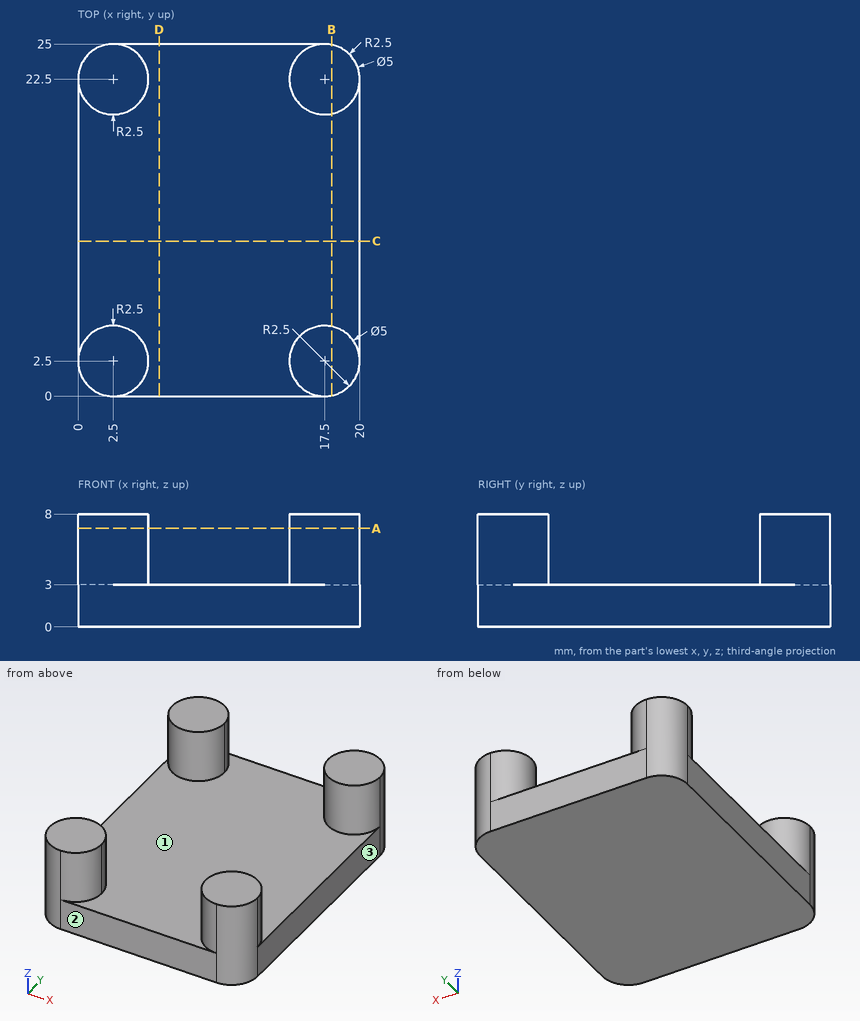
Study the drawing (mm; zero at the part's minimum x, y, z) and answer. Coordinates: 2 decimals unless noted, no trailing zeros. Write each loop counter-clockwise with the first axis right and the second up, starting at its lowest first coordinate (ties: lowest second). Pieces come first, ordered by that corner, then holes.
Q1. A cutting plane is placed at C-C, the plane y = 11. Give the vertices of the cut face in (x, z).
Q2. A cutting plane is placed at B-B, the plane x = 18. Give the vertices of the cut face in (y, z), then the cut area to 3 significant figures.
Q3. Determine the mould class of the marked faces 1, 2 and 3 for opening direction Y: released by +Y, released by -Y, zero draft, split by the parting line, or undercut.
Q4. Each of these flat-tipped pins is pushed along its axis until it touches: pin 1 Ø1 at (x, y) = (5, 21) entering from +Z; pin 2 Ø1 at (x, z) = (11, 4.5) entering from -Y; pin 3 Ø3 at (x, y) = (11, 5.5) entering from +Z. Where does it stop, or does it pass through?
Q5. A cutting plane is placed at D-D, the plane x = 5.75. Give the vertices of the cut face in (y, z).
Q6. A cutting plane is placed at A-A, the plane z = 7. Give the vertices of the cut face in (x, y), then the cut area to 3 significant figures.
Q7. Find the intervals of material crossed by line 1 (Z direction, x = 8.5, y = 17); line 2 (Y direction, x = 3, z = 6); line 3 (Y direction, x = 2.75, z = 7.75), in increasing order.
Findings below:
1. outline: (0, 0) - (20, 0) - (20, 3) - (0, 3) - close
2. outline: (0.05, 0) - (24.95, 0) - (24.95, 8) - (20.05, 8) - (20.05, 3) - (4.95, 3) - (4.95, 8) - (0.05, 8) - close
2. area: 124 mm2
3. face 1: undercut
3. face 2: released by -Y
3. face 3: zero draft
4. pin 1: stops at z = 8
4. pin 2: passes through
4. pin 3: stops at z = 3
5. outline: (0, 0) - (25, 0) - (25, 3) - (0, 3) - close
6. outline: circle Ø5 at (2.5, 2.5); circle Ø5 at (2.5, 22.5); circle Ø5 at (17.5, 2.5); circle Ø5 at (17.5, 22.5)
6. area: 78.5 mm2
7. line 1: z = 0 to 3
7. line 2: y = 0.05 to 4.95, 20.05 to 24.95
7. line 3: y = 0.01 to 4.99, 20.01 to 24.99
